Can you work these out from the model? Positions are in its coordinate system, mm. Face numbers are marked on the shaded views. Round coordinates to 2 decimals unless told otherwise and drop trailing zeros. Loops run counter-clockwise (first coordinate to the right, second up) from the corner with the lowest first, then second, coordinate; pieces in that order, holes last.
(1) I want a section at C-C on x = 7.25. Write out the boundary of the cut face in (y, z), plus the area to 3 significant figures.
(2) I want a section at A-A on x = -6. Write out the boundary of the cut face in (y, z), plus the area to 3 significant figures.
(3) Will these pins go through, and if not, where does the flat tip stop? pin 1 Ø4 at (x, z) = (2, 10.5) entering from +Y; pin 2 Ø8 at (x, y) = (5.5, -3) entering from -Z; pin 3 Ø3 at (x, z) = (1, 10) entering from -Y; pin 4 Ø6 at (y, z) = (-1, 2) entering from -X.
(4) Thinking about a two-plate mould opening in Y: for the marked faces 1, 2 and 3, which applies, released by +Y, released by -Y, zero draft, split by the parting line, or undercut?
(5) I want a section at B-B on z = -35. Write out the boundary of the cut face in (x, y) (3 decimals), plus the area to 3 significant figures.
(6) If I drill on line 1 along X through (y, z) = (0, 12.5); line 2 along Z through (x, y) = (6.75, -3); line 3 along Z through (x, y) = (3.75, 0.75), over which ranges is the centre line in solid material (lowest first)?
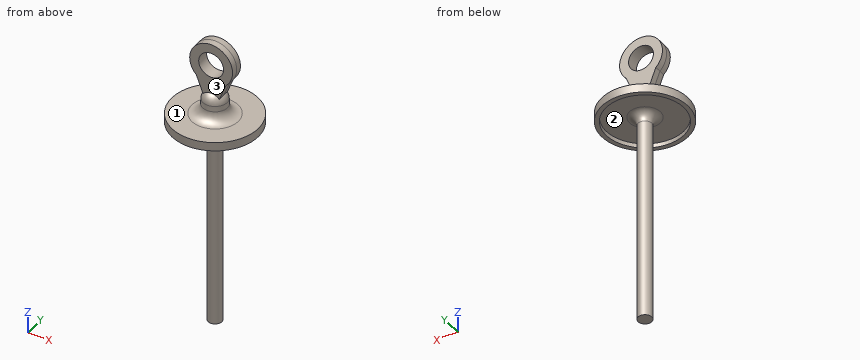
from build123d import *

# Parameters (mm, degrees)
SKETCH1_R                     = 3
BASE_EXTRUDE_DEPTH            = 6
BASE_EXTRUDE_TAPER            = 3
FILLET1_R                     = 2.5
BOSS_EXTRUDE1_DEPTH           = 1.45
BOSS_EXTRUDE1_TAPER           = 2
BOSS_EXTRUDE1_OTHER_WAY_DEPTH = 1.45
BOSS_EXTRUDE1_OTHER_WAY_TAPER = 2
SKETCH3_R                     = 2.9
CUT_EXTRUDE1_DEPTH            = 19.796475854
SKETCH4_R                     = 1.585
BOSS_EXTRUDE2_DEPTH           = 50
SKETCH5_R                     = 10
SKETCH5_R_2                   = 1.585
BOSS_EXTRUDE3_DEPTH           = 1
SKETCH11_R                    = 10
SKETCH11_R_2                  = 9
EXTRUDE1_DEPTH                = 1
FILLET5_R                     = 2.5
FILLET6_R                     = 2


with BuildPart() as part:
    # Sketch1 → Base-Extrude (new body)
    with BuildSketch(Plane.XY):
        Circle(SKETCH1_R)
    extrude(amount=BASE_EXTRUDE_DEPTH, taper=BASE_EXTRUDE_TAPER)

    # Fillet1
    fillet1_edges = [part.edges().sort_by_distance(p)[0] for p in [
        (-2.685553324, 0, 6),
    ]]
    fillet(fillet1_edges, radius=FILLET1_R)

    # Sketch2 → Boss-Extrude1 (add)
    with BuildSketch(Plane(origin=(0, 0, 0), x_dir=(1, 0, 0), z_dir=(0, 1, 0))):
        with BuildLine():
            Line((3.495897193, -8.85566154), (0, 0))
            Line((0, 0), (-3.495897193, -8.85566154))
            ThreePointArc((-3.495897193, -8.85566154), (0, -17.55), (3.495897193, -8.85566154))
        make_face()
    extrude(amount=BOSS_EXTRUDE1_DEPTH, taper=BOSS_EXTRUDE1_TAPER)

    # Sketch2 → Boss-Extrude1 other way (add)
    with BuildSketch(Plane(origin=(0, 0, 0), x_dir=(1, 0, 0), z_dir=(0, 1, 0))):
        with BuildLine():
            Line((3.495897193, -8.85566154), (0, 0))
            Line((0, 0), (-3.495897193, -8.85566154))
            ThreePointArc((-3.495897193, -8.85566154), (0, -17.55), (3.495897193, -8.85566154))
        make_face()
    extrude(amount=-BOSS_EXTRUDE1_OTHER_WAY_DEPTH, taper=BOSS_EXTRUDE1_OTHER_WAY_TAPER)

    # Sketch3 → Cut-Extrude1 (cut, through all)
    with BuildSketch(Plane.XZ.offset(1.45)):
        with Locations(Location((0, 12.5, 0), (0, 0, 270))):
            Circle(SKETCH3_R)
    extrude(amount=-CUT_EXTRUDE1_DEPTH, mode=Mode.SUBTRACT)

    # Sketch4 → Boss-Extrude2 (add)
    with BuildSketch(Plane(origin=(0, 0, 0), x_dir=(-1, 0, 0), z_dir=(0, 0, -1))):
        with Locations(Location((0, 0, 0), (0, 0, 180))):
            Circle(SKETCH4_R)
    extrude(amount=BOSS_EXTRUDE2_DEPTH)

    # Sketch5 → Boss-Extrude3 (add)
    with BuildSketch(Plane(origin=(0, 0, 0), x_dir=(-1, 0, 0), z_dir=(0, 0, -1))):
        Circle(SKETCH5_R)
        Circle(SKETCH5_R_2, mode=Mode.SUBTRACT)
    extrude(amount=BOSS_EXTRUDE3_DEPTH)

    # Sketch11 → Extrude1 (add)
    with BuildSketch(Plane(origin=(0, 0, -1), x_dir=(-1, 0, 0), z_dir=(0, 0, -1))):
        Circle(SKETCH11_R)
        Circle(SKETCH11_R_2, mode=Mode.SUBTRACT)
    extrude(amount=EXTRUDE1_DEPTH)

    # Fillet5
    fillet5_edges = [part.edges().sort_by_distance(p)[0] for p in [
        (-3, 0, 0),
    ]]
    fillet(fillet5_edges, radius=FILLET5_R)

    # Fillet6
    fillet6_edges = [part.edges().sort_by_distance(p)[0] for p in [
        (-1.585, 0, -1),
    ]]
    fillet(fillet6_edges, radius=FILLET6_R)


solid = part.part
Filled sheet:
1. outline: (-6.89, -2) - (-5.33, -2) - (-5.33, -1) - (5.33, -1) - (5.33, -2) - (6.89, -2) - (6.89, 0) - (-6.89, 0) - close
1. area: 16.9 mm2
2. outline: (-8, -2) - (-6.71, -2) - (-6.71, -1) - (6.71, -1) - (6.71, -2) - (8, -2) - (8, 0) - (-8, 0) - close
2. area: 18.6 mm2
3. pin 1: stops at y = 1.45
3. pin 2: stops at z = -2
3. pin 3: stops at y = -1.45
3. pin 4: stops at x = -10
4. face 1: zero draft
4. face 2: undercut
4. face 3: released by -Y
5. outline: circle Ø3.17 at (0, 0)
5. area: 7.89 mm2
6. line 1: x = -5.05 to -2.9, 2.9 to 5.05
6. line 2: z = -1 to 0
6. line 3: z = -1 to 0.54, 9.16 to 15.84
